```python
from build123d import *

# Parameters (mm, degrees)
PAD_DEPTH        = 60
THICKNESS_T      = 3
SKETCH001_W      = 25
SKETCH001_H      = 3
PAD001_DEPTH     = 40
HOLE_D           = 3.4
HOLE_DEPTH       = 12
HOLE_CBORE_D     = 6
HOLE_CBORE_DEPTH = 0.5
FILLET_R         = 7


with BuildPart() as part:
    # Sketch → Pad (new body)
    with BuildSketch(Plane.XY):
        with BuildLine():
            ThreePointArc((-12.5, 37.99671), (0, -40), (12.5, 37.99671))
            Line((-12.5, 37.99671), (12.5, 37.99671))
        make_face()
    extrude(amount=PAD_DEPTH)

    # Thickness
    thickness_openings = [part.faces().sort_by_distance(p)[0] for p in [
        (0, -0.260782, 60),
    ]]
    offset(amount=THICKNESS_T, openings=thickness_openings)

    # Sketch001 (on Face4 of Thickness) → Pad001 (join)
    with BuildSketch(Plane.XY.offset(60)):
        with Locations((0, 39.49671)):
            Rectangle(SKETCH001_W, SKETCH001_H)
    extrude(amount=PAD001_DEPTH)

    # Hole
    with Locations(Plane.XZ.offset(-37.99671)):
        with Locations((-5.5, 93), (5.5, 93)):
            CounterBoreHole(HOLE_D / 2, HOLE_CBORE_D / 2, HOLE_CBORE_DEPTH, depth=HOLE_DEPTH)

    # Fillet
    fillet_edges = [part.edges().sort_by_distance(p)[0] for p in [
        (12.5, 39.49671, 100),
        (-12.5, 39.49671, 100),
    ]]
    fillet(fillet_edges, radius=FILLET_R)


solid = part.part
```
Can you work these out from the model? Positions are in its coordinate system, mm. A direction names the side the tool comes from. Round coordinates to 2 decimals unless told otherwise and drop trailing zeros. Loops run counter-clockwise (first coordinate to the right, second up) from the corner with the lowest first, then second, coordinate; pieces in that order, holes last. Notation, with made-up numbers: (-8.75, -27) -> (30.25, -27) arc R18 cw to (30.25, 5) -> close; hole circle Ø6 at (78, 1.5). An arc over 180 degrees is marked (long way). One line per item, written item: value. Start each with the question number.
1. For faces 4 (the flat face through (-12.5, 39, 76)), 5 (the flat face through (12.5, 39, 76)), 6 (the cylindrical face through (-6.15, 38.24, 90.07)), 7 (the flat face through (0, 37.997, 49)), which set-ups out of +Z, -Z, +X, -X, +Y, -Y let a thin tool reach every point of the face, with its end or its side?
2. If I drill on probe 1 along X at (y, z) = (39, 93); probe 2 along Y at (x, z) = (0, 35.5); probe 3 along Z at (x, y) = (-12.5, 2), over which ranges is the centre line in solid material (lowest first)?
3. If we section it at A-A, the plane z = 31: Write out the boundary of the cut face in (x, y).
4. For pin 1 (4 mm diameter, centred on y = -3.5, z = 25.5, fed in from +X); pin 2 (0.9 mm diameter, centred on y = 39, z = 84.5, fed in from +X); pin 3 (20 mm diameter, centred on x = -4, z = 66, fed in from -Y), each with a flat end and sliding along its axis, tell me the tip position at first contact or that it passes through.
5. If we mould it in two halves opening along Y, with no side actions, what happens to faces 1 (the cylindrical face through (-1.699, -42.966, 29.58)), 2 (the cylindrical face through (-5.13, 39.76, 91.34)), 3 (the flat face through (-1, 0, 0))? For each: pulls with the +Y half, pulls with the -Y half, needs draft (parallel to the pull), parting line crosses it, or undercut.
Calculated:
1. face 4: +Z, -X, +Y, -Y
1. face 5: +Z, +X, +Y, -Y
1. face 6: -Y
1. face 7: +Z
2. probe 1: x = -12.5 to -7.2, -3.8 to 3.8, 7.2 to 12.5
2. probe 2: y = -43 to -40, 38 to 41
2. probe 3: z = -3 to 0
3. outline: (-13.44, 40.85) arc R43 ccw (long way) to (13.44, 40.85) arc R3 ccw to (12.5, 41) -> (-12.5, 41) arc R3 ccw to start; hole (-12.5, 38) arc R40 ccw (long way) to (12.5, 38) -> close
4. pin 1: stops at x = 42.97
4. pin 2: stops at x = 12.5
4. pin 3: stops at y = -43
5. face 1: parting line crosses it
5. face 2: needs draft
5. face 3: undercut
